Geometry check sheet. Reference: the model listing, model coordinates, mm. A direction names the side the tool comes from. Give positions to 0.01 mm unless a question says otherwise; leave off trailing zeros. Loops run counter-clockwise (first coordinate to the right, second up) from the corner with the lowest first, then second, coordinate; pieces in that order, holes last.
```python
from build123d import *

# Parameters (mm, degrees)
F1_DEPTH = 20
F2_R     = 2.125
F3_DEPTH = 12
F4_R     = 2.125
F5_DEPTH = 1.5
F6_R     = 3.5
F7_R     = 1


with BuildPart() as f1:
    # F0 (on Front) → F1 (new body)
    with BuildSketch(Plane.XZ):
        Polygon((-12.5, 16.5), (-12.5, 11.75), (-12.5, 9.25), (-12.5, 7.5), (-12.5, 4.5), (12.5, 4.5), (12.5, 7.5), (-10, 7.5), (-10, 13.5), (12.5, 13.5), (12.5, 16.5), align=None)
    extrude(amount=F1_DEPTH)

    # F2 (on face) → F3 (cut, through all)
    with BuildSketch(Plane.XY.offset(16.5)):
        with Locations((0.625, -10)):
            Circle(F2_R)
    extrude(amount=-F3_DEPTH, mode=Mode.SUBTRACT)

    # F4 (on face) → F5 (cut)
    with BuildSketch(Plane.XY.offset(16.5)):
        Polygon((2.9344010768, -14), (5.2438021535, -10), (2.9344010768, -6), (-1.6844010768, -6), (-3.9938021535, -10), (-1.6844010768, -14), align=None)
        with Locations((0.625, -10)):
            Circle(F4_R, mode=Mode.SUBTRACT)
    extrude(amount=-F5_DEPTH, mode=Mode.SUBTRACT)

    # F6
    f6_edges = [f1.edges().sort_by_distance(p)[0] for p in [
        (-12.5, -10, 4.5),
        (-12.5, -10, 16.5),
    ]]
    fillet(f6_edges, radius=F6_R)

    # F7
    f7_edges = [f1.edges().sort_by_distance(p)[0] for p in [
        (-10, -10, 13.5),
        (-10, -10, 7.5),
        (12.5, -10, 7.5),
        (12.5, -10, 13.5),
        (-9, -10, 4.5),
        (-9, -10, 16.5),
        (12.5, -10, 4.5),
        (12.5, -10, 16.5),
    ]]
    fillet(f7_edges, radius=F7_R)


solid = f1.part
```
1) Depth check by flat-ended pin: P1, Ø4, axis at x = 0.625, y = -10, coming from the -Z side; P2, Ø1.2, axis at y = -12.5, z = 10.5, coming from the +X side. Enter the tip coordinate at first touch or a pass-through.
2) Sectioned sample at A-A on x = -7.75. Enter the section's corners in (y, z).
3) Tool access check on faces 4 (the flat face through (-2.82, -7.97, 15.76)), 5 (the cylindrical face through (-11.5, -10.14, 5.55)), 6 (the cylindrical face through (-9.699, -10.14, 7.785)). Record the directions out of +Z, -Z, +X, -X, +Y, -Y that give a thin tool (end or side, any length) a straight path to the whole face; none if there is none.
4) Sectioned sample at B-B on y = -17. Enter the section's corners in (x, z), plus the area to 3 significant figures.
5) Scan lines: line 1 along Z through (x, y) = (11, -10); line 2 along Z through (x, y) = (-3.5, -10.75); line 3 along X through (y, z) = (-13.5, 11.5). Record each from-to range of solid material in increasing order.
6) Sectioned sample at C-C on x = 1.25. Enter the section's corners in (y, z), plus the area to 3 significant figures.
7) Sectioned sample at D-D on z = 11.25. Enter the section's corners in (x, y).
8) Mould release check, pull along Z, two halves, no side actions. Record for faces 1 (the flat face through (0, -20, 7)), 2 (the cylindrical face through (12.215, -10.14, 13.801)), 3 (the flat face through (3, -9, 15)): +Z half, -Z half, draft (parallel to the pull), parting line (faces both ways), or undercut.
Determined:
1. P1: passes through
1. P2: stops at x = -10
2. outline: (-20, 4.5) - (0, 4.5) - (0, 7.5) - (-20, 7.5) - close; (-20, 13.5) - (0, 13.5) - (0, 16.5) - (-20, 16.5) - close
3. face 4: +Z
3. face 5: -Z, -X, +Y, -Y
3. face 6: +X, +Y, -Y
4. outline: (-12.5, 8) arc R3.5 ccw to (-9, 4.5) - (11.5, 4.5) arc R1 ccw to (12.5, 5.5) - (12.5, 6.5) arc R1 ccw to (11.5, 7.5) - (-9, 7.5) arc R1 cw to (-10, 8.5) - (-10, 12.5) arc R1 cw to (-9, 13.5) - (11.5, 13.5) arc R1 ccw to (12.5, 14.5) - (12.5, 15.5) arc R1 ccw to (11.5, 16.5) - (-9, 16.5) arc R3.5 ccw to (-12.5, 13) - close
4. area: 159 mm2
5. line 1: z = 4.5 to 7.5, 13.5 to 16.5
5. line 2: z = 4.5 to 7.5, 13.5 to 15
5. line 3: x = -12.5 to -10
6. outline: (-20, 4.5) - (-12.03, 4.5) - (-12.03, 7.5) - (-20, 7.5) - close; (-20, 13.5) - (-12.03, 13.5) - (-12.03, 15) - (-14, 15) - (-14, 16.5) - (-20, 16.5) - close; (-7.97, 4.5) - (0, 4.5) - (0, 7.5) - (-7.97, 7.5) - close; (-7.97, 13.5) - (0, 13.5) - (0, 16.5) - (-6, 16.5) - (-6, 15) - (-7.97, 15) - close
6. area: 89.7 mm2
7. outline: (-12.5, -20) - (-10, -20) - (-10, 0) - (-12.5, 0) - close
8. face 1: draft
8. face 2: undercut
8. face 3: +Z half
